```python
from build123d import *

# Parameters (mm, degrees)
SKETCH1_R           = 1.375
BOSS_EXTRUDE1_DEPTH = 1
SKETCH2_W           = 50.9
SKETCH2_H           = 5
SKETCH2_W_2         = 7.8
SKETCH2_H_2         = 4.8
SKETCH2_W_3         = 11.2
SKETCH2_H_3         = 6.5
SKETCH2_W_4         = 12
SKETCH2_H_4         = 13
SKETCH2_H_5         = 12
CUT_EXTRUDE1_DEPTH  = 0.01


with BuildPart() as part:
    # Sketch1 → Boss-Extrude1 (new body)
    with BuildSketch(Plane.XY):
        with BuildLine():
            Line((29.5, -15), (-29.5, -15))
            ThreePointArc((-29.5, -15), (-31.621320344, -14.121320344), (-32.5, -12))
            Line((-32.5, -12), (-32.5, 12))
            ThreePointArc((-32.5, 12), (-31.621320344, 14.121320344), (-29.5, 15))
            Line((-29.5, 15), (29.5, 15))
            ThreePointArc((29.5, 15), (31.621320344, 14.121320344), (32.5, 12))
            Line((32.5, 12), (32.5, -12))
            ThreePointArc((32.5, -12), (31.621320344, -14.121320344), (29.5, -15))
        make_face()
        with Locations((-29, 11.5)):
            Circle(SKETCH1_R, mode=Mode.SUBTRACT)
        with Locations((-29, -11.5)):
            Circle(SKETCH1_R, mode=Mode.SUBTRACT)
        with Locations((29, -11.5)):
            Circle(SKETCH1_R, mode=Mode.SUBTRACT)
        with Locations((29, 11.5)):
            Circle(SKETCH1_R, mode=Mode.SUBTRACT)
    extrude(amount=BOSS_EXTRUDE1_DEPTH)

    # Sketch2 → Cut-Extrude1 (cut)
    with BuildSketch(Plane.XY.offset(1)):
        with Locations((0, 11.5)):
            Rectangle(SKETCH2_W, SKETCH2_H)
        with Locations((21.5, -12.6)):
            Rectangle(SKETCH2_W_2, SKETCH2_H_2)
        with Locations((8.9, -12.6)):
            Rectangle(SKETCH2_W_2, SKETCH2_H_2)
        with Locations((-20.1, -11.75)):
            Rectangle(SKETCH2_W_3, SKETCH2_H_3)
        with Locations((-21, 1.9)):
            Rectangle(SKETCH2_W_4, SKETCH2_H_4)
        with Locations((-3.5, -2)):
            Rectangle(SKETCH2_W_4, SKETCH2_H_5)
    extrude(amount=-CUT_EXTRUDE1_DEPTH, mode=Mode.SUBTRACT)


solid = part.part
```
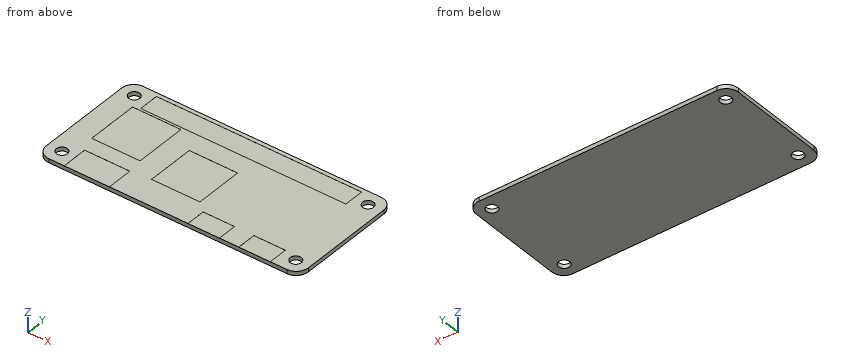
Here's how the part is built. I have some questions about the finished solid (model axes, mm). Coordinates: 2 decimals unless noted, no trailing zeros. Order: outer loops, then holes, each group sorted by start corner. A loop starts at its lowest first (then second) coordinate and runs counter-clockwise, first axis right, second up. Notation, with made-up numbers: (12, -37.75) -> (39, -37.75) arc R33 cw to (39, 1.25) -> close; hole circle Ø1 at (-10.75, 70.5). An arc over 180 degrees is marked (long way). Return JSON: item names as keys, results as strings.
1) If I drill on probe 1 along Y at (x, z) = (29, 0.6) (3 decimals); probe 2 along Z at (x, y) = (-17, 11.5), over which ranges is the centre line in solid material (lowest first)?
Conclusion:
{"probe 1": "y = -15 to -12.875, -10.125 to 10.125, 12.875 to 15", "probe 2": "z = 0 to 0.99"}
2) I'm going to push a flat-ended pin straight in: P1, Ø1.4, axis at x = 23.5, y = -12.5, coming from the +Z side. Where does the tip first touch, or does it pass through?
Conclusion:
{"P1": "stops at z = 0.99"}
3) If we section it at A-A on z = 0.55: List the corners of the cut face in (x, y) for me (3 decimals), plus the area to 3 significant figures.
Conclusion:
{"outline": "(-32.5, -12) arc R3 ccw to (-29.5, -15) -> (29.5, -15) arc R3 ccw to (32.5, -12) -> (32.5, 12) arc R3 ccw to (29.5, 15) -> (-29.5, 15) arc R3 ccw to (-32.5, 12) -> close; hole circle Ø2.75 at (-29, -11.5); hole circle Ø2.75 at (-29, 11.5); hole circle Ø2.75 at (29, -11.5); hole circle Ø2.75 at (29, 11.5)", "area": "1,920 mm²"}
